Source: three-view drawing plus pictorial views. Frame: mm from the lowest corner of the part. A direction names the side the tool comes from. Coordinates: 2 decimals unless noted, no trailing zeros. Write each loop counter-clockwise with the first axis right and the second up, starting at its lowest first coordinate (ties: lowest second). Pieces come first, ordered by that corner, then holes. Notation, with made-up numbers: (-15.75, 19) - (5.25, 19) arc R33 cw to (5.25, 56) - close; hole circle Ø4 at (63, 64.5). An arc over 180 degrees is marked (long way). One line per item, written item: value.
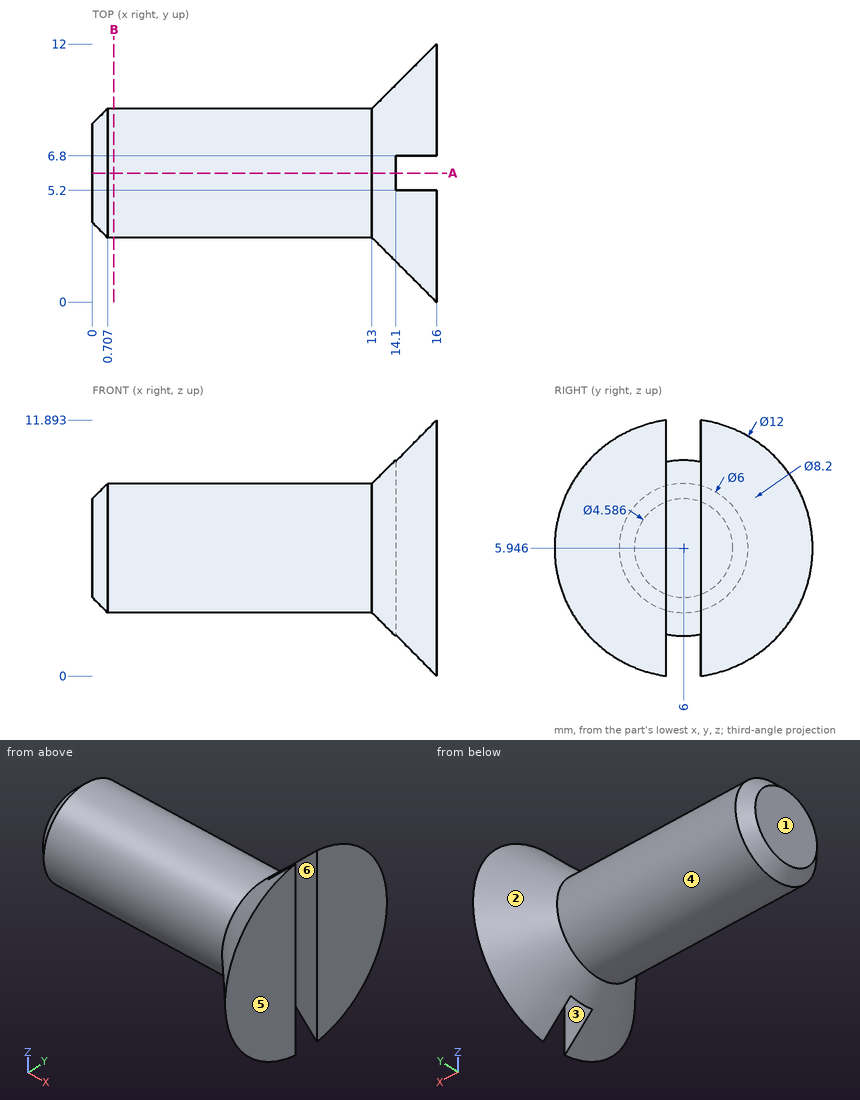
1) Contact query for flat-ended pins moving along their axis: P1, Ø6, axis at x = 9, z = 2.5, coming from the +Y side; P2, Ø6, axis at x = 5.5, y = 8.5, coming from the -Z side; P3, Ø1, axis at x = 15, z = 8, coming from the -Y side (1 decimal). Output: stop coordinate, or through.
Values found:
P1: y = 8.97
P2: z = 2.95
P3: y = 0.9
2) Section query B-B on x = 1. Output: boundary loops of the cut face in (y, z).
Values found:
outline: circle Ø6 at (6, 5.95)
3) Draft query along Y for the marked faces 1, 2 and 3. Return one class per face: released by +Y, released by -Y, zero draft, split by the parting line, or undercut.
Values found:
face 1: zero draft
face 2: split by the parting line
face 3: undercut
4) Material intervals for line 1 (Y direction, x = 14.25, z = 6.5) (1 decimal); line 2 (Y direction, x = 4, z = 8.25); line 3 (Y direction, x = 14.75, z = 3.25), sorted ascending.
Values found:
line 1: 1.8 to 5.2, 6.8 to 10.2
line 2: 4.08 to 7.92
line 3: 2.09 to 5.2, 6.8 to 9.91
5) Reachability of the marked faces 4, 5 and 6 from +Z, -Z, +X, -X, +Y, -Y: full face, straight path, thin tool, end or side. Return the list, or none.
Values found:
face 4: -X
face 5: +Z, -Z, +X, +Y, -Y
face 6: +Z, -Z, +X
6) Section query A-A on y = 6. Output: boundary loops of the cut face in (x, z), then the cut area to 3 significant figures.
Values found:
outline: (0, 3.65) - (0.71, 2.95) - (13, 2.95) - (14.1, 1.85) - (14.1, 10.05) - (13, 8.95) - (0.71, 8.95) - (0, 8.24) - close
area: 85.3 mm2
